Source: CAD feature listing. Evaluate the final solid. Frame: model axes, mm. Face numbers are marked on the shaded views. Give positions to 0.01 mm unless a question says otherwise; leave off trailing zeros. Order: outer loops, then holes, each group sorted by start corner. A loop starts at its lowest first (then second) coordinate and runs counter-clockwise, first axis right, second up. Notation, with made-up numbers: M -35,61 L 10,61 A12 cw 10,78 Z; hole C 37,72.25 d7. An arc over 180 degrees is marked long. Use CSV: the item, a comma, the result in double quotes. Start each with the question number.
Item 1: First-contact query: pin 1 (1.5 mm diameter, centred on x = 1, z = 1, fed in from +Y); pin 2 (2.5 mm diameter, centred on y = 0, z = 0, fed in from +X). Flat tips, straight axial feed; report the tip coordinate or a pass-through.
Item 2: Section query A-A on y = 0. Return loops of the section in (x, z).
Item 3: Pull-direction query (Z, two-part tool) for the marked faces 1, 2, 3 and 4; classes: +Z half, -Z half, draft (parallel to the pull), parting line (faces both ways), or undercut.
Item 4: Section query D-D on x = 2.25. Return loops of the section in (y, z).
Item 5: Ray query, probe 1 along Y at (x, z) = (0.5, 0); probe 2 along Y at (x, z) = (2.3, -0.25); probe 3 along Z at (x, y) = (2.9, -0.5). Return the intervals inside material, ascending. Write a range as from..to.
Item 6: Section query C-C on x = 1.3. Return loops of the section in (y, z).
Autodesk Inventor part; units mm, degrees
ref_plane "YZ Plane" through (0, 0, 0) normal (1, 0, 0) x (0, 1, 0)
ref_plane "XZ Plane" through (0, 0, 0) normal (0, 1, 0) x (-1, 0, 0)
ref_plane "XY Plane" through (0, 0, 0) normal (0, 0, 1) x (1, 0, 0)
sketch "スケッチ1" plane through (0, 0, 0) normal (1, 0, 0) x (0, 1, 0)
  circle A0 centre (0, 0) radius 3.5
  dimension "d0" = 7
extrude "押し出し1" add sketch "スケッチ1" along normal blind 4
sketch "スケッチ2" plane through (4, 0, 0) normal (1, 0, 0) x (0, 0, -1)
  circle A0 centre (0, 0) radius 2
  dimension "d3" = 4
extrude "押し出し2" cut sketch "スケッチ2" against normal blind 2
sketch "スケッチ3" plane through (0, 0, 0) normal (-1, 0, 0) x (0, 0, 1)
  circle A0 centre (0, 0) radius 1.5
  dimension "d6" = 3
extrude "押し出し3" cut sketch "スケッチ3" against normal blind 2
chamfer "面取り1" distance 1 angle 45 1 edges at (0, -3.5, 0)
properties part number "MagnetStopper"
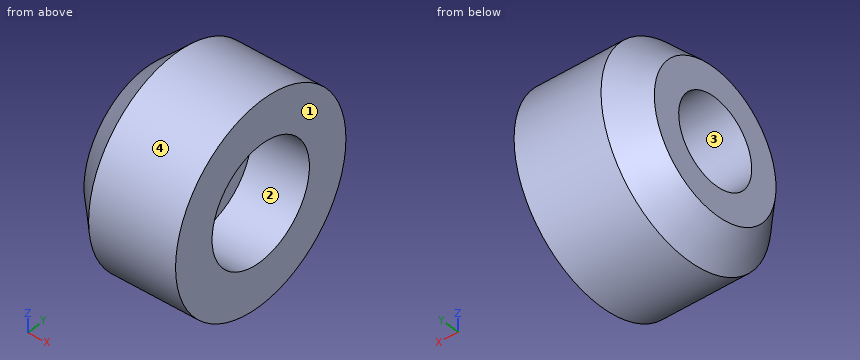
Verdict:
1,pin 1,"y = 3.49"
1,pin 2,"through"
2,outline,"M 0,-2.5 L 1,-3.5 L 4,-3.5 L 4,-2 L 2,-2 L 2,-1.5 L 0,-1.5 Z; M 0,1.5 L 2,1.5 L 2,2 L 4,2 L 4,3.5 L 1,3.5 L 0,2.5 Z"
3,face 1,"draft"
3,face 2,"undercut"
3,face 3,"undercut"
3,face 4,"parting line"
4,outline,"C 0,0 d7; hole C 0,0 d4"
5,probe 1,"-3..-1.5, 1.5..3"
5,probe 2,"-3.49..-1.98, 1.98..3.49"
5,probe 3,"-3.46..-1.94, 1.94..3.46"
6,outline,"C 0,0 d7; hole C 0,0 d3"
